Read the model definition and answer for the solid it produces. Units are mm, in the model's axes. A direction names the side the tool comes from. Coordinates: 2 decimals unless noted, no trailing zeros. Write each loop counter-clockwise with the first axis right and the second up, starting at its lowest first coordinate (ties: lowest second). Pieces come first, ordered by that corner, then holes. Notation, with made-up numbers: (-2, 77.5) -> (22, 77.5) arc R11 ccw to (22, 93.5) -> close; hole circle Ø4 at (28, -5.5). An arc over 180 degrees is marked (long way). Use CSV: the item, a comma, the result in double quotes.
from build123d import *

# Parameters (mm, degrees)
SKETCH1_W               = 100
SKETCH1_H               = 100
BOSS_EXTRUDE1_DEPTH     = 10
SKETCH2_R               = 3.25
CUT_EXTRUDE1_DEPTH      = 10
SKETCH3_OUTSIDE_W       = 130.354
SKETCH3_OUTSIDE_H       = 130.354
SKETCH3_OUTSIDE_R       = 50
CUT_EXTRUDE2_DEPTH      = 10
SKETCH4_R               = 2.5
CUT_EXTRUDE3_DEPTH      = 10
SKETCH5_R               = 3.25
CUT_EXTRUDE4_DEPTH      = 10
SKETCH6_R               = 6.25
CUT_EXTRUDE5_DEPTH      = 5
SKETCH7_R               = 15
BOSS_EXTRUDE2_DEPTH     = 5
CHAMFER1_SIZE           = 2
SKETCH8_R               = 41
SKETCH8_R_2             = 27
CUT_EXTRUDE_THIN1_DEPTH = 4


with BuildPart() as part:
    # Sketch1 → Boss-Extrude1 (new body)
    with BuildSketch(Plane(origin=(0, 0, 0), x_dir=(1, 0, 0), z_dir=(0, 1, 0))):
        Rectangle(SKETCH1_W, SKETCH1_H)
    extrude(amount=BOSS_EXTRUDE1_DEPTH)

    # Sketch2 → Cut-Extrude1 (cut)
    with BuildSketch(Plane(origin=(0, 10, 0), x_dir=(1, 0, 0), z_dir=(0, 1, 0))):
        with Locations(Location((-25, 0, 0), (0, 0, 270))):
            Circle(SKETCH2_R)
        with Locations(Location((0, 25, 0), (0, 0, 270))):
            Circle(SKETCH2_R)
        with Locations(Location((25, 0, 0), (0, 0, 270))):
            Circle(SKETCH2_R)
        with Locations(Location((0, -25, 0), (0, 0, 270))):
            Circle(SKETCH2_R)
    extrude(amount=-CUT_EXTRUDE1_DEPTH, mode=Mode.SUBTRACT)

    # Sketch3 outside → Cut-Extrude2 (cut)
    with BuildSketch(Plane(origin=(0, 10, 0), x_dir=(1, 0, 0), z_dir=(0, 1, 0))):
        Rectangle(SKETCH3_OUTSIDE_W, SKETCH3_OUTSIDE_H)
        with Locations(Location((0, 0, 0), (0, 0, 270))):
            Circle(SKETCH3_OUTSIDE_R, mode=Mode.SUBTRACT)
    extrude(amount=-CUT_EXTRUDE2_DEPTH, mode=Mode.SUBTRACT)

    # Sketch4 → Cut-Extrude3 (cut)
    with BuildSketch(Plane(origin=(0, 10, 0), x_dir=(1, 0, 0), z_dir=(0, 1, 0))):
        with Locations(Location((-31.819805153, 31.819805153, 0), (0, 0, 270))):
            Circle(SKETCH4_R)
        with Locations(Location((31.819805153, 31.819805153, 0), (0, 0, 270))):
            Circle(SKETCH4_R)
        with Locations(Location((31.819805153, -31.819805153, 0), (0, 0, 270))):
            Circle(SKETCH4_R)
        with Locations(Location((-31.819805153, -31.819805153, 0), (0, 0, 270))):
            Circle(SKETCH4_R)
    extrude(amount=-CUT_EXTRUDE3_DEPTH, mode=Mode.SUBTRACT)

    # Sketch5 → Cut-Extrude4 (cut)
    with BuildSketch(Plane.XZ):
        with Locations(Location((-22.273863607, 22.273863607, 0), (0, 0, 270))):
            Circle(SKETCH5_R)
        with Locations(Location((22.273863607, -22.273863607, 0), (0, 0, 270))):
            Circle(SKETCH5_R)
    extrude(amount=-CUT_EXTRUDE4_DEPTH, mode=Mode.SUBTRACT)

    # Sketch6 → Cut-Extrude5 (cut)
    with BuildSketch(Plane.XZ):
        with Locations(Location((25, 0, 0), (0, 0, 270))):
            Circle(SKETCH6_R)
        with Locations(Location((22.273863607, -22.273863607, 0), (0, 0, 270))):
            Circle(SKETCH6_R)
        with Locations(Location((0, -25, 0), (0, 0, 270))):
            Circle(SKETCH6_R)
        with Locations(Location((-25, 0, 0), (0, 0, 270))):
            Circle(SKETCH6_R)
        with Locations(Location((-22.273863607, 22.273863607, 0), (0, 0, 270))):
            Circle(SKETCH6_R)
        with Locations(Location((0, 25, 0), (0, 0, 270))):
            Circle(SKETCH6_R)
    extrude(amount=-CUT_EXTRUDE5_DEPTH, mode=Mode.SUBTRACT)

    # Sketch7 → Boss-Extrude2 (add)
    with BuildSketch(Plane(origin=(0, 10, 0), x_dir=(1, 0, 0), z_dir=(0, 1, 0))):
        with Locations(Location((0, 0, 0), (0, 0, 90))):
            Circle(SKETCH7_R)
    extrude(amount=BOSS_EXTRUDE2_DEPTH)

    # Chamfer1
    chamfer1_edges = [part.edges().sort_by_distance(p)[0] for p in [
        (0, 15, 15),
    ]]
    chamfer(chamfer1_edges, length=CHAMFER1_SIZE)

    # Sketch8 → Cut-Extrude-Thin1 (cut)
    with BuildSketch(Plane.XZ):
        Circle(SKETCH8_R)
        Circle(SKETCH8_R_2, mode=Mode.SUBTRACT)
    extrude(amount=-CUT_EXTRUDE_THIN1_DEPTH, mode=Mode.SUBTRACT)


solid = part.part
1. For a pull along X with two mould halves and no side action, classify faces 3 (the cylindrical face through (30.86, 5.07, -29.51)), 4 (the flat face through (10, 10, -12)) as pulls with the +X half, pulls with the -X half, needs draft (parallel to the pull), parting line crosses it, or undercut.
Solutions:
face 3,"undercut"
face 4,"needs draft"
2. A tool of negligible diameter and unlimited length cuts with its end or side. For faces 1 (the cylindrical face through (-17.004, 3.576, 18.914)), 2 (the cylindrical face through (-33.341, 5.07, 29.836)), from which of +Z, -Z, +X, -X, +Y, -Y can it reach the whole face along a straight path? Write none if from no direction.
Solutions:
face 1,"-Y"
face 2,"+Y, -Y"
3. Find the intervals of material crossed by line 1 along X through (y, z) = (8.55, 0); line 2 along X through (y, z) = (3.25, -24); line 3 along Z through (x, y) = (1, 7.25), in increasing order.
Solutions:
line 1,"x = -50 to -28.25, -21.75 to 21.75, 28.25 to 50"
line 2,"x = -43.86 to -33.24, -12.37 to -6.17, 6.17 to 12.37, 33.24 to 43.86"
line 3,"z = -49.99 to -28.09, -21.91 to 21.91, 28.09 to 49.99"
4. Each of these flat-tipped pins is pushed along its axis until it touches: pin 1 Ø10 at (x, z) = (-22.27, 22.27) entering from +Y; pin 2 Ø6 at (x, z) = (0, 24) entering from -Y; pin 3 Ø4 at (x, z) = (0, 25) entering from -Y; pin 4 Ø10 at (x, z) = (-20, 20) entering from -Y. Where does it stop, or does it pass through?
Solutions:
pin 1,"stops at y = 10"
pin 2,"stops at y = 5"
pin 3,"passes through"
pin 4,"stops at y = 0"
5. A cutting plane is placed at C-C (y = 1.75). Give the vertices of the cut face in (x, z), and give its area (3 significant figures).
Solutions:
outline,"circle Ø100 at (0, 0); (-26.3, -6.11) arc R27 ccw to (-6.11, -26.3) arc R6.25 cw (long way) to (6.11, -26.3) arc R27 ccw to (16.05, -21.71) arc R6.25 cw to (21.71, -16.05) arc R27 ccw to (26.3, -6.11) arc R6.25 cw (long way) to (26.3, 6.11) arc R27 ccw to (6.11, 26.3) arc R6.25 cw (long way) to (-6.11, 26.3) arc R27 ccw to (-16.05, 21.71) arc R6.25 cw to (-21.71, 16.05) arc R27 ccw to (-26.3, 6.11) arc R6.25 cw (long way) to start; hole circle Ø82 at (0, 0); hole circle Ø5 at (-31.82, -31.82); hole circle Ø5 at (-31.82, 31.82); hole circle Ø5 at (31.82, -31.82); hole circle Ø5 at (31.82, 31.82)"
area,"4,430 mm^2"
6. A cutting plane is placed at A-A (z = 0). Give the number of separate pieces and of enclosed holes in the cut face, and give its area (3 significant figures).
Solutions:
separate pieces,"3"
enclosed holes,"0"
area,"878 mm^2"
